The listing builds one solid part. Answer for the finished solid, in the listing's coordinates (mm). Face numbers are marked on the shaded views. A direction names the side the tool comes from. Round coordinates to 2 decimals unless told otherwise and drop trailing zeros. Write each loop counter-clockwise with the first axis right and the second up, starting at its lowest first coordinate (ties: lowest second). Pieces come first, ordered by that corner, then holes. Notation, with made-up numbers: (78, 34.25) - (131, 34.25) arc R20 cw to (131, 50.25) - close; hole circle Ø1 at (-13.5, 85). An arc over 180 degrees is marked (long way). Answer in a Markdown table with one row per item.
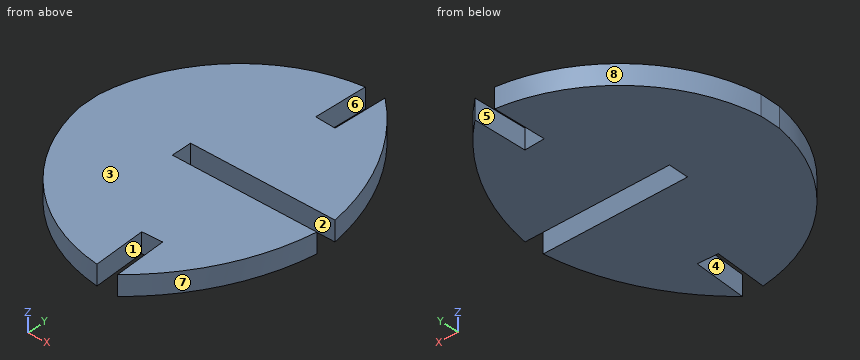
from build123d import *

# Parameters (mm, degrees)
BOSS_EXTRUDE1_DEPTH = 1.524


with BuildPart() as part:
    # Sketch1 → Boss-Extrude1 (new body)
    with BuildSketch(Plane.XY):
        with BuildLine():
            Line((68.053425724, 0), (68.053425724, -1.524))
            Line((68.053425724, -1.524), (78.95165892, -1.524))
            ThreePointArc((78.95165892, -1.524), (77.077407117, -7.264754764), (73.322018867, -11.994040562))
            Line((73.322018867, -11.994040562), (73.141160104, -8.002049555))
            Line((73.141160104, -8.002049555), (71.618721766, -8.071024238))
            Line((71.618721766, -8.071024238), (71.798167573, -12.031827879))
            ThreePointArc((71.798167573, -12.031827879), (64.673060187, -8.599062053), (61.138299457, -1.524))
            Line((61.138299457, -1.524), (61.138299457, 0))
            ThreePointArc((61.138299457, 0), (64.673060187, 7.075062053), (71.798167573, 10.507827879))
            Line((71.798167573, 10.507827879), (71.618721766, 6.547024238))
            Line((71.618721766, 6.547024238), (73.141160104, 6.478049555))
            Line((73.141160104, 6.478049555), (73.322018867, 10.470040562))
            ThreePointArc((73.322018867, 10.470040562), (77.077407117, 5.740754764), (78.95165892, 0))
            Line((78.95165892, 0), (68.053425724, 0))
        make_face()
    extrude(amount=BOSS_EXTRUDE1_DEPTH)


solid = part.part
(1) Section A-A (y = -9.75) is taken. Give the vertices of the cut face in (x, z).
Checked values:
| item | result |
|---|---|
| outline | (66.02, 0) - (71.69, 0) - (71.69, 1.52) - (66.02, 1.52) - close; (73.22, 0) - (75.45, 0) - (75.45, 1.52) - (73.22, 1.52) - close |
(2) Section D-D (y = -6.25) is taken. Give the vertices of the cut face in (x, z).
Checked values:
| item | result |
|---|---|
| outline | (62.81, 0) - (77.58, 0) - (77.58, 1.52) - (62.81, 1.52) - close |
(3) Flat-ended cylindrical pins translate along their axes: pin 1 (0.5 mm diameter, centred on x = 72.5, z = 0.5, fed in from -Y); pin 2 (0.8 mm diameter, centred on y = -1, z = 1, fed in from +X). Find the tip coordinate at first contact, or state that the pin passes through.
Checked values:
| item | result |
|---|---|
| pin 1 | stops at y = -8.04 |
| pin 2 | stops at x = 68.05 |
(4) Section B-B (z = 0.5) is taken. Give the vertices of the cut face in (x, y).
Checked values:
| item | result |
|---|---|
| outline | (61.14, -1.52) arc R12.23 ccw to (71.8, -12.03) - (71.62, -8.07) - (73.14, -8) - (73.32, -11.99) arc R17.07 ccw to (78.95, -1.52) - (68.05, -1.52) - (68.05, 0) - (78.95, 0) arc R17.07 ccw to (73.32, 10.47) - (73.14, 6.48) - (71.62, 6.55) - (71.8, 10.51) arc R12.23 ccw to (61.14, 0) - close |
(5) Section C-C (x = 71) is taken. Give the vertices of the cut face in (y, z), and give its area (3 significant figures).
Checked values:
| item | result |
|---|---|
| outline | (-11.91, 0) - (-1.52, 0) - (-1.52, 1.52) - (-11.91, 1.52) - close; (0, 0) - (10.38, 0) - (10.38, 1.52) - (0, 1.52) - close |
| area | 31.7 mm2 |
(6) Find the intervals of material crossed by line 1 (X direction, y = 7, z = 0.65); line 2 (Y direction, x = 74, z = 0.3); line 3 (Y direction, x = 74.5, z = 0.85), in increasing order.
Checked values:
| item | result |
|---|---|
| line 1 | x = 64.6 to 71.64, 73.16 to 76.33 |
| line 2 | y = -11.36 to -1.52, 0 to 9.84 |
| line 3 | y = -10.85 to -1.52, 0 to 9.33 |
(7) For the marked faces 1, 2, 3, 4 and 5, determine the directions among +Z, -Z, +X, -X, +Y, -Y from which every point of the face is accessible in a straight line to the end or side of a thin tool.
Checked values:
| item | result |
|---|---|
| face 1 | +Z, -Z |
| face 2 | +Z, -Z, +X |
| face 3 | +Z, +X, -X, +Y, -Y |
| face 4 | +Z, -Z, -Y |
| face 5 | +Z, -Z, +Y |
(8) For a pull along X with two mould halves and no side action, classify the marked faces 6, 7 and 8 as pulls with the +X half, pulls with the -X half, needs draft (parallel to the pull), parting line crosses it, or undercut.
Checked values:
| item | result |
|---|---|
| face 6 | undercut |
| face 7 | pulls with the +X half |
| face 8 | pulls with the -X half |
